For this review, take the finished solid that the model builds, in its own axes (mm). A direction names the side the tool comes from. Coordinates: 2 decimals unless noted, no trailing zeros. Order: outer loops, then holes, each group sorted by start corner. A loop starts at its lowest first (then second) coordinate and runs counter-clockwise, first axis right, second up. Notation, with made-up numbers: (40.5, 66.5) -> (95.5, 66.5) arc R12 ccw to (95.5, 76.5) -> close; hole circle Ø6 at (52, 37.25). An arc over 180 degrees is marked (long way). Return JSON: item names as keys, results as strings. Group by question number.
Item 1: For line 1 along Z through (x, y) = (15, -0.75); line 2 along X through (y, z) = (6.5, 7.5); line 3 along Y through (x, z) = (1.5, 6), list the stretches that pass through material, from the lowest coordinate up.
Item 2: Draft analysis for pull direction Y (two halves, no side actions). For faces 1 (the flat face through (30, 8, 7)), 2 (the flat face through (29, 25, 5)), 3 (the cylindrical face through (-8.458, 48.387, 1.531)), state which applies: +Y half, -Y half, draft (parallel to the pull), parting line (faces both ways), or undercut.
Item 3: Machinability: for faces 4 (the cylindrical face through (43.5, 1.56, 3.93)), 5 (the flat face through (8.199, 49.605, 1.233)), 6 (the flat face through (51.199, 49.605, 3.767)), which of the approach directions +Z, -Z, +X, -X, +Y, -Y give a long, thin tool a straight path to every point of the face, cutting with its end or side? Answer none if there is none.
Item 4: Take a section at B-B (x = 6.5). Write out the cut boundary in (y, z).
Item 5: Take a section at D-D (x = 45). Write out the cut boundary in (y, z).
Item 6: Insertion check: pin 1 (10 mm diameter, centred on x = 14, y = 22.5, fed in from -Z); pin 2 (2.5 mm diameter, centred on x = 45, z = 4, fed in from -Y); pin 3 (4 mm diameter, centred on x = 64.5, z = 2, fed in from -Y); pin 4 (0.8 mm diameter, centred on x = 56, z = 4.5, fed in from +Y). Each pin has a flat end and moves straight along its axis. Give the tip position at first contact, or say it passes through.
Item 7: Take a section at A-A (y = 5). Write out the cut boundary in (x, z), then the cut area to 3 significant figures.
Item 8: Take a section at C-C (y = 30.5). Write out the cut boundary in (x, z), then the cut area to 3 significant figures.
Autodesk Inventor part; units mm, degrees
ref_plane "YZ Plane" through (0, 0, 0) normal (1, 0, 0) x (0, 1, 0)
ref_plane "XZ Plane" through (0, 0, 0) normal (0, 1, 0) x (-1, 0, 0)
ref_plane "XY Plane" through (0, 0, 0) normal (0, 0, 1) x (1, 0, 0)
sketch "스케치1" plane through (0, 0, 0) normal (0, 0, 1) x (1, 0, 0)
  line L0 (0, 0) -> (60, 0)
  line L1 (60, 0) -> (60, 25)
  line L2 (60, 57) -> (0, 57)
  line L3 (0, 25) -> (0, 0)
  line L4 (-13, 57) -> (73, 57)
  line L5 (73, 57) -> (73, 25)
  line L6 (-13, 25) -> (-13, 57)
  line L7 (73, 25) -> (60, 25)
  line L8 (0, 25) -> (-13, 25)
  dimension "d0" = 60
  dimension "d1" = 57
  dimension "d3" = 86
  dimension "d4" = 32
  dimension "d5" = 13
extrude "돌출1" add sketch "스케치1" along normal blind 8
sketch "스케치2" plane through (0, 0, 8) normal (0, 0, 1) x (1, 0, 0)
  line L0 (0, 0) -> (60, 0)
  line L1 (60, 0) -> (60, 25)
  line L2 (60, 25) -> (73, 25)
  line L3 (73, 25) -> (73, 57)
  line L4 (73, 57) -> (-13, 57)
  line L5 (-13, 57) -> (-13, 25)
  line L6 (-13, 25) -> (0, 25)
  line L7 (0, 25) -> (0, 0)
  line L8 (0, 25) -> (0, 0)
  line L9 (0, 8) -> (60, 8)
  line L10 (60, 8) -> (60, 0)
  line L11 (60, 0) -> (0, 0)
  line L12 (0, 0) -> (0, 8)
  dimension "d9" = 8
  dimension "d10" = 0
extrude "돌출2" cut sketch "스케치2" against normal blind 3 contours L7 L6 L5 L4 L3 L2 L1 L9
sketch "스케치4" plane through (0, 0, 0) normal (0, -1, 0) x (1, 0, 0)
  line L0 (0, 0) -> (60, 0)
  line L1 (60, 0) -> (60, 8)
  line L2 (0, 8) -> (60, 8)
  line L3 (0, 0) -> (0, 8)
  circle A0 centre (45, 4) radius 1.5
  circle A1 centre (15, 4) radius 1.5
  dimension "d15" = 3
  dimension "d16" = 3
  dimension "d17" = 4
  dimension "d18" = 15
  dimension "d19" = 4
  dimension "d20" = 15
extrude "돌출4" cut sketch "스케치4" against normal blind 6 contours A0 | A1
sketch "스케치11" plane through (-13, 57, 5) normal (0, 1, 0) x (1, 0, 0)
  line L0 (0, 0) -> (86, 0)
  line L1 (86, 5) -> (86, 0)
  line L2 (86, 5) -> (0, 5)
  line L3 (0, 5) -> (0, 0)
  line L4 (0, 2.5) -> (43, 0)
  line L5 (0, 0) -> (86, 0)
  line L6 (73, 5) -> (86, 5)
  line L7 (43, 0) -> (43, 2.5)
  line L8 (86, 5) -> (0, 5)
  line L9 (86, 5) -> (43, 2.5)
  line L10 (0, 5) -> (43, 2.5)
  line L11 (43, 0) -> (86, 2.5)
  line L12 (86, 5) -> (86, 0)
  line L13 (86, 2.5) -> (86, 5)
  point P0 (13, 5)
extrude "돌출7" cut sketch "스케치11" against normal blind 15 contours L3 L4 L0 | L11 L1 L0 | L10 L2 L9
sketch "스케치13" plane through (-13, 57, 2.5) normal (-0.058, 0, 0.9983) x (0.9983, 0, 0.058)
  circle A0 centre (3, -8) radius 1.6
  circle A1 centre (40, -8) radius 1.6
  line L0 (0, -15) -> (0, 0)
  line L1 (0, 0) -> (43.0726, 0)
  line L2 (42.9275, -15) -> (-0.1451, -15)
  point P0 (12.833, -57)
  dimension "d53" = 3.2
  dimension "d54" = 3.2
  dimension "d55" = 37
  dimension "d56" = 3
  dimension "d57" = 8
  dimension "d58" = 7
extrude "돌출8" cut sketch "스케치13" against normal blind 3
sketch "스케치15" plane through (0, 0, 0) normal (0, -1, 0) x (1, 0, 0)
  circle A0 centre (45, 4) radius 1.5
  circle A1 centre (15, 4) radius 1.5
  line L0 (0, 0) -> (60, 0)
  line L1 (60, 0) -> (60, 8)
  line L2 (0, 8) -> (60, 8)
  line L3 (0, 0) -> (0, 8)
extrude "돌출11" add sketch "스케치15" along normal blind 3
sketch "스케치16" plane through (30, 42, 5) normal (0.058, 0, 0.9983) x (0.9983, 0, -0.058)
  circle A0 centre (40.0726, 7) radius 1.6
  circle A1 centre (3.0737, 7.28) radius 1.6
  line L0 (0, 15) -> (43.0726, 15)
  line L1 (43.0726, 15) -> (43.0726, 0)
  point P0 (-29.6592, -42)
  dimension "d71" = 3.2
  dimension "d72" = 3.2
  dimension "d73" = 8
  dimension "d74" = 7.72
  dimension "d75" = 37
  dimension "d76" = 3
extrude "돌출12" cut sketch "스케치16" against normal blind 10
properties part number "앞뒷면PSD받침대_수정" material "ABS 플라스틱"
Findings below:
{
 "1": {"line 1": "z = 0 to 2.5, 5.5 to 8", "line 2": "x = 0 to 60", "line 3": "y = -3 to 8"},
 "2": {"face 1": "+Y half", "face 2": "draft", "face 3": "undercut"},
 "3": {"face 4": "-Y", "face 5": "-Z, +Y", "face 6": "+Z, +X, +Y"},
 "4": {"outline": "(-3, 0) -> (42, 0) -> (42, 1.13) -> (57, 1.13) -> (57, 3.63) -> (42, 3.63) -> (42, 5) -> (8, 5) -> (8, 8) -> (-3, 8) -> close"},
 "5": {"outline": "(-3, 0) -> (42, 0) -> (42, 1.63) -> (57, 1.63) -> (57, 4.13) -> (42, 4.13) -> (42, 5) -> (8, 5) -> (8, 8) -> (-3, 8) -> (-3, 5.5) -> (6, 5.5) -> (6, 2.5) -> (-3, 2.5) -> close"},
 "6": {"pin 1": "stops at z = 0", "pin 2": "stops at y = 6", "pin 3": "stops at y = 25", "pin 4": "stops at y = 42"},
 "7": {"outline": "(0, 0) -> (60, 0) -> (60, 8) -> (0, 8) -> close; hole circle Ø3 at (15, 4); hole circle Ø3 at (45, 4)", "area": "466 mm2"},
 "8": {"outline": "(-13, 0) -> (73, 0) -> (73, 5) -> (-13, 5) -> close", "area": "430 mm2"}
}
